```python
from build123d import *

# Parameters (mm, degrees)
SKETCH1_W                                        = 756
SKETCH1_H                                        = 15
BOSS_EXTRUDE1_DEPTH                              = 15
CUT_EXTRUDE1_DEPTH                               = 757.185989027
CUT_EXTRUDE2_DEPTH                               = 757.185989027
DRAFT1_ANGLE                                     = 45
DRAFT2_ANGLE                                     = 45
HOLE1_D                                          = 3.1199998
CBORE_FOR_M4_HEX_HEAD_MACHINE_SCREW1_D           = 4.5
CBORE_FOR_M4_HEX_HEAD_MACHINE_SCREW1_CBORE_D     = 7.5
CBORE_FOR_M4_HEX_HEAD_MACHINE_SCREW1_CBORE_DEPTH = 5.3
CHAMFER1_SIZE                                    = 0.359114068
CHAMFER2_SIZE                                    = 0.351583128
CHAMFER2_SIZE_2                                  = 0.314005893
CHAMFER3_SIZE                                    = 0.348386014
CHAMFER4_SIZE                                    = 0.699992786
CHAMFER4_SIZE2                                   = 0.69999271
CHAMFER5_SIZE                                    = 0.69999271
CHAMFER5_SIZE2                                   = 0.699992786


with BuildPart() as part:
    # Sketch1 → Boss-Extrude1 (new body)
    with BuildSketch(Plane(origin=(0, 15, 0), x_dir=(-1, 0, 0), z_dir=(0, 1, 0))):
        with Locations((238, 0)):
            Rectangle(SKETCH1_W, SKETCH1_H)
    extrude(amount=-BOSS_EXTRUDE1_DEPTH)

    # Sketch2 → Cut-Extrude1 (cut, through all)
    with BuildSketch(Plane.ZY.offset(616)):
        with BuildLine():
            Line((-7.5, 11.135189072), (-7.5, 4.2000246))
            Line((-7.5, 4.2000246), (-4.8000183, 4.2000246))
            Line((-4.8000183, 4.2000246), (-4.8000183, 8.8400054))
            Line((-4.8000183, 8.8400054), (-5.754192018, 9.794179118))
            ThreePointArc((-5.754192018, 9.794179118), (-6.350212567, 10.82514773), (-7.5, 11.135189072))
        make_face()
    extrude(amount=-CUT_EXTRUDE1_DEPTH, mode=Mode.SUBTRACT)

    # Sketch3 → Cut-Extrude2 (cut, through all)
    with BuildSketch(Plane.ZY.offset(616)):
        with BuildLine():
            Line((7.5, 4.2000246), (7.5, 11.135189072))
            ThreePointArc((7.5, 11.135189072), (6.350212567, 10.82514773), (5.754192018, 9.794179118))
            Line((5.754192018, 9.794179118), (4.8000183, 8.8400054))
            Line((4.8000183, 8.8400054), (4.8000183, 4.2000246))
            Line((4.8000183, 4.2000246), (7.5, 4.2000246))
        make_face()
    extrude(amount=-CUT_EXTRUDE2_DEPTH, mode=Mode.SUBTRACT)

    # Draft1
    draft1_faces = [part.faces().sort_by_distance(p)[0] for p in [
        (-238, 4.2000246, -6.15000915),
    ]]
    draft(draft1_faces, Plane(origin=(140, 0, -7.5), x_dir=(-1, 0, 0), z_dir=(0, 0, -1)), DRAFT1_ANGLE)

    # Draft2
    draft2_faces = [part.faces().sort_by_distance(p)[0] for p in [
        (-238, 4.2000246, 6.15000915),
    ]]
    draft(draft2_faces, Plane(origin=(-616, 0, 7.5), x_dir=(1, 0, 0), z_dir=(0, 0, 1)), DRAFT2_ANGLE)

    # Hole1 (through all)
    with Locations(Plane.ZY.offset(616)):
        with Locations((-7.3005066, 14.813004), (7.3005066, 14.813004)):
            Hole(HOLE1_D / 2)

    # CBORE for M4 Hex Head Machine Screw1 (through all)
    with Locations(Plane(origin=(0, 15, 0), x_dir=(-1, 0, 0), z_dir=(0, 1, 0))):
        with Locations((-60, 0), (-120, 0), (0, 0), (60, 0), (120, 0), (180, 0), (240, 0), (300, 0), (360, 0), (420, 0), (480, 0), (540, 0), (600, 0)):
            CounterBoreHole(CBORE_FOR_M4_HEX_HEAD_MACHINE_SCREW1_D / 2, CBORE_FOR_M4_HEX_HEAD_MACHINE_SCREW1_CBORE_D / 2, CBORE_FOR_M4_HEX_HEAD_MACHINE_SCREW1_CBORE_DEPTH)

    # Chamfer1
    # the kernel refuses this chamfer: 0.359114068, 0.320732608 mm, written as the material it takes off along each edge
    with BuildSketch(Plane(origin=(-616.923527515, 13.265812328, 7.5), x_dir=(0, -1, 0), z_dir=(1, 0, 0))) as chamfer1_piece_1:
        with BuildLine():
            Line((CHAMFER1_SIZE * 0.99999999892, 0), (0.005140565, 0.353974179))
            ThreePointArc((0.005140565, 0.353974179), (0.01270895, 0.181894047), (0, 0))
            Line((0, 0), (CHAMFER1_SIZE * 0.99999999892, 0))
        make_face()
    extrude(amount=757.84705503, mode=Mode.SUBTRACT)
    with BuildSketch(Plane(origin=(-616.923527515, 13.265812328, -7.5), x_dir=(0, -0.014520899519340609, 0.9998945661804294), z_dir=(1, 0, 0))) as chamfer1_piece_2:
        with BuildLine():
            Line((0.354011504, 0), (CHAMFER1_SIZE * 0.0145208995037, CHAMFER1_SIZE * 0.999894565101))
            Line((CHAMFER1_SIZE * 0.0145208995037, CHAMFER1_SIZE * 0.999894565101), (0, 0))
            ThreePointArc((0, 0), (0.182059415, 0.010066344), (0.354011504, 0))
        make_face()
    extrude(amount=757.84705503, mode=Mode.SUBTRACT)

    # Chamfer2
    # the kernel refuses this chamfer: 0.351583128, 0.314005893 mm, written as the material it takes off along each edge
    with BuildSketch(Plane(origin=(-616.904160355, 11.135189072, -7.5), x_dir=(0, 0.017205827635516736, 0.9998519687910691), z_dir=(1, 0, 0))) as chamfer2_piece_1:
        with BuildLine():
            Line((0.345686311, 0), (CHAMFER2_SIZE * 0.0172058276427, -CHAMFER2_SIZE * 0.999851969207))
            Line((CHAMFER2_SIZE * 0.0172058276427, -CHAMFER2_SIZE * 0.999851969207), (0, 0))
            ThreePointArc((0, 0), (0.177775336, -0.009597014), (0.345686311, 0))
        make_face()
    extrude(amount=757.808320711, mode=Mode.SUBTRACT)
    with BuildSketch(Plane(origin=(-617.049666566, 11.135189072, 7.5), x_dir=(0, 1, 0), z_dir=(1, 0, 0))) as chamfer2_piece_2:
        with BuildLine():
            Line((CHAMFER2_SIZE_2 * 0.999999998673, 0), (-0.001272129, -0.408616458))
            ThreePointArc((-0.001272129, -0.408616458), (0.012772883, -0.209994562), (0, 0))
            Line((0, 0), (CHAMFER2_SIZE_2 * 0.999999998673, 0))
        make_face()
    extrude(amount=758.099333132, mode=Mode.SUBTRACT)

    # Chamfer3
    # the kernel refuses this chamfer: 0.348386014, 0.313117398 mm, written as the material it takes off along each edge
    with BuildSketch(Plane(origin=(-616.895938121, 15, 5.751754785), x_dir=(0, 0, -1), z_dir=(1, 0, 0))) as chamfer3_piece_1:
        with BuildLine():
            Line((CHAMFER3_SIZE, 0), (0.003206731, -0.345186893))
            ThreePointArc((0.003206731, -0.345186893), (0.011218763, -0.177431259), (0, 0))
            Line((0, 0), (CHAMFER3_SIZE, 0))
        make_face()
    extrude(amount=757.791876243, mode=Mode.SUBTRACT)
    with BuildSketch(Plane(origin=(-616.895938121, 15, -5.751754785), x_dir=(0, 0, 1), z_dir=(1, 0, 0))) as chamfer3_piece_2:
        with BuildLine():
            Line((CHAMFER3_SIZE, 0), (0.003206731, 0.345186893))
            ThreePointArc((0.003206731, 0.345186893), (0.011218763, 0.177431259), (0, 0))
            Line((0, 0), (CHAMFER3_SIZE, 0))
        make_face()
    extrude(amount=757.791876243, mode=Mode.SUBTRACT)

    # Chamfer4
    chamfer4_edges = [part.edges().sort_by_distance(p)[0] for p in [
        (-238, 0, 7.5),
    ]]
    chamfer4_side = [part.faces().sort_by_distance(p)[0] for p in [
        (-238, 2.1000123, 7.5),
    ]]
    chamfer(chamfer4_edges, length=CHAMFER4_SIZE, length2=CHAMFER4_SIZE2, reference=chamfer4_side[0])

    # Chamfer5
    chamfer5_edges = [part.edges().sort_by_distance(p)[0] for p in [
        (-238, 0, -7.5),
    ]]
    chamfer5_side = [part.faces().sort_by_distance(p)[0] for p in [
        (-608.438647672, 0, -0.349996355),
    ]]
    chamfer(chamfer5_edges, length=CHAMFER5_SIZE, length2=CHAMFER5_SIZE2, reference=chamfer5_side[0])


solid = part.part
```
For this review, take the finished solid that the model builds, in its own axes (mm). Give positions to 0.01 mm unless a question says otherwise; leave off trailing zeros. Loops run counter-clockwise (first coordinate to the right, second up) from the corner with the lowest first, then second, coordinate; pieces in that order, holes last. Notation, with made-up numbers: M 7.5,-3 L 52.5,-3 A16 ccw 52.5,8 Z; hole C 73.25,-28 d7. An arc over 180 degrees is marked long. One line per item, written item: value. Start each with the question number.
Q1. Clearance check with flat-ended pins moving along their axes: pin 1 Ø6 at (x, y) = (-412.5, 7.5) entering from -Z; pin 2 Ø4 at (x, z) = (-358.5, -1.5) entering from +Y; pin 3 Ø1.5 at (x, y) = (-456.5, 7) entering from -Z; pin 4 Ø4 at (x, z) = (-181.5, -0.5) entering from +Y. State where each tip first meets the part, or that it passes through.
Q2. Add section B-B (z = 0). Count the separate pieces of the cut face and the enclosed holes in it, and give its area (3 significant figures).
Q3. Add section A-A (x = -337). Give the boundary of the cut face in (y, z).
Q4. For L1, parallel to Z at x = -240, y = 7.5; L2, parallel to Z at x = -240, y = 6.25; L3, parallel to Z at x = -456.5, y = 8, list the stretches that pass through material, from the lowest coordinate up.
Reply:
1. pin 1: z = -7.2
1. pin 2: y = 15
1. pin 3: z = -5.45
1. pin 4: y = 9.7
2. separate pieces: 14
2. enclosed holes: 0
2. area: 10,300 mm²
3. outline: M 0,-6.8 L 0.7,-7.5 L 4.2,-7.5 L 6.9,-4.8 L 8.84,-4.8 L 9.79,-5.75 A1.56 cw 11.14,-7.15 L 11.49,-7.5 L 12.91,-7.5 L 13.26,-7.15 A1.56 cw 14.65,-5.75 L 15,-5.4 L 15,5.4 L 14.65,5.75 A1.56 cw 13.26,7.15 L 12.91,7.5 L 11.45,7.5 L 11.13,7.09 A1.56 cw 9.79,5.75 L 8.84,4.8 L 6.9,4.8 L 4.2,7.5 L 0.7,7.5 L 0,6.8 Z
4. L1: -4.8 to -2.25, 2.25 to 4.8
4. L2: -5.45 to -2.25, 2.25 to 5.45
4. L3: -4.8 to 4.8
